```python
from build123d import *

# Parameters (mm, degrees)
F0_W     = 25
F0_H     = 48
F0_R     = 1
F0_W_2   = 12.5
F0_H_2   = 23
F1_DEPTH = 4.25
F2_R     = 6


with BuildPart() as f1:
    # F0 (on Top) → F1 (new body)
    with BuildSketch(Plane.XY):
        with Locations((0, -5.5)):
            Rectangle(F0_W, F0_H)
        with Locations((0, -13.75)):
            Circle(F0_R, mode=Mode.SUBTRACT)
        Rectangle(F0_W_2, F0_H_2, mode=Mode.SUBTRACT)
        with Locations((0, 13.75)):
            Circle(F0_R, mode=Mode.SUBTRACT)
    extrude(amount=F1_DEPTH)

    # F2
    f2_edges = [f1.edges().sort_by_distance(p)[0] for p in [
        (-12.5, 18.5, 2.125),
        (12.5, 18.5, 2.125),
        (12.5, -29.5, 2.125),
        (-12.5, -29.5, 2.125),
    ]]
    fillet(f2_edges, radius=F2_R)


solid = f1.part
```
Verification items for the finished model (mm, model axes). A direction names the side the tool comes from. Give positions to 0.01 mm unless a question says otherwise; leave off trailing zeros. Order: outer loops, then holes, each group sorted by start corner. A loop starts at its lowest first (then second) coordinate and runs counter-clockwise, first axis right, second up. Notation, with made-up numbers: (-11, 58) - (24, 58) arc R31 ccw to (24, 82) - close; hole circle Ø8 at (27, 11.5). An arc over 180 degrees is marked (long way). Answer as CSV lines item,"result". Start each with the question number.
Item 1: Access from +Z, -Z, +X, -X, +Y, -Y to the whole of each face (thin tool, end or side, straight path). Record for faces 5 (the face through (0, -11.5, 2)), 6 (the face through (0, -16, 0)).
Item 2: Section check C-C, the plane x = -3.25. Record the boundary of the cut face in (y, z).
Item 3: Mould release check, pull along Y, two halves, no side actions. Record for faces 1 (the face through (-0.217, 12.774, 2.095)), 2 (the face through (0, 18.5, 2)), 3 (the face through (-12.5, -6, 2)), 4 (the face through (0, -29.5, 2)): released by +Y, released by -Y, zero draft, split by the parting line, or undercut.
Item 4: Section check D-D, the plane z = 0.95. Record the boundary of the cut face in (x, y), plus the area to 3 significant figures.
Item 5: Material ranges on L1, parallel to Y at x = 0, z = 1.95; L2, parallel to Y at x = 5.25, z = 0.4; L3, parallel to X at y = 6.5, z = 0.5, recorded low to high.
Item 6: Section check B-B, the plane y = -13.75. Record the boundary of the cut face in (x, z), plus the area to 4 significant figures.
Item 7: Section check A-A, the plane x = 0. Record the boundary of the cut face in (y, z), plus the area to 4 significant figures.
Filled in:
1,face 5,"+Z, -Z"
1,face 6,"-Z, +X, -X, +Y, -Y"
2,outline,"(-29.5, 0) - (-11.5, 0) - (-11.5, 4.25) - (-29.5, 4.25) - close; (11.5, 0) - (18.5, 0) - (18.5, 4.25) - (11.5, 4.25) - close"
3,face 1,"undercut"
3,face 2,"released by +Y"
3,face 3,"zero draft"
3,face 4,"released by -Y"
4,outline,"(-12.5, -23.5) arc R6 ccw to (-6.5, -29.5) - (6.5, -29.5) arc R6 ccw to (12.5, -23.5) - (12.5, 12.5) arc R6 ccw to (6.5, 18.5) - (-6.5, 18.5) arc R6 ccw to (-12.5, 12.5) - close; hole (-6.25, -11.5) - (6.25, -11.5) - (6.25, 11.5) - (-6.25, 11.5) - close; hole circle Ø2 at (0, -13.75); hole circle Ø2 at (0, 13.75)"
4,area,"875 mm^2"
5,L1,"-29.5 to -14.75, -12.75 to -11.5, 11.5 to 12.75, 14.75 to 18.5"
5,L2,"-29.5 to -11.5, 11.5 to 18.5"
5,L3,"-12.5 to -6.25, 6.25 to 12.5"
6,outline,"(-12.5, 0) - (-1, 0) - (-1, 4.25) - (-12.5, 4.25) - close; (1, 0) - (12.5, 0) - (12.5, 4.25) - (1, 4.25) - close"
6,area,"97.75 mm^2"
7,outline,"(-29.5, 0) - (-14.75, 0) - (-14.75, 4.25) - (-29.5, 4.25) - close; (-12.75, 0) - (-11.5, 0) - (-11.5, 4.25) - (-12.75, 4.25) - close; (11.5, 0) - (12.75, 0) - (12.75, 4.25) - (11.5, 4.25) - close; (14.75, 0) - (18.5, 0) - (18.5, 4.25) - (14.75, 4.25) - close"
7,area,"89.25 mm^2"
